from build123d import *

# Parameters (mm, degrees)
SKETCH1_R           = 88.9
SKETCH1_R_2         = 2.1
BOSS_EXTRUDE1_DEPTH = 6.35
SKETCH2_R           = 57.3
CUT_EXTRUDE1_DEPTH  = 3


with BuildPart() as part:
    # Sketch1 → Boss-Extrude1 (new, symmetric)
    with BuildSketch(Plane.XY):
        Circle(SKETCH1_R)
        with Locations((-12, 0)):
            Circle(SKETCH1_R_2, mode=Mode.SUBTRACT)
        with Locations((-6, 10.392304845)):
            Circle(SKETCH1_R_2, mode=Mode.SUBTRACT)
        with Locations((6, 10.392304845)):
            Circle(SKETCH1_R_2, mode=Mode.SUBTRACT)
        with Locations((12, 0)):
            Circle(SKETCH1_R_2, mode=Mode.SUBTRACT)
        with Locations((6, -10.392304845)):
            Circle(SKETCH1_R_2, mode=Mode.SUBTRACT)
        with Locations((-6, -10.392304845)):
            Circle(SKETCH1_R_2, mode=Mode.SUBTRACT)
    extrude(amount=BOSS_EXTRUDE1_DEPTH, both=True)

    # Sketch2 → Cut-Extrude1 (cut)
    with BuildSketch(Plane(origin=(0, 0, -6.35), x_dir=(-1, 0, 0), z_dir=(0, 0, -1))):
        Circle(SKETCH2_R)
    extrude(amount=-CUT_EXTRUDE1_DEPTH, mode=Mode.SUBTRACT)


solid = part.part
Design review of the part built by this model. Coordinates are the model's own, in mm. A direction names the side the tool comes from. Coordinates: 2 decimals unless noted, no trailing zeros. Write each loop counter-clockwise with the first axis right and the second up, starting at its lowest first coordinate (ties: lowest second). Pieces come first, ordered by that corner, then holes. Notation, with made-up numbers: (60, 46.5) - (101, 46.5) arc R11 cw to (101, 62.5) - close; hole circle Ø9 at (20, -9). An arc over 180 degrees is marked (long way). One line per item, written item: value.
1) Add section B-B (x = 0). State the section outline as (y, z) points.
Answer sheet:
outline: (-88.9, -6.35) - (-57.3, -6.35) - (-57.3, -3.35) - (57.3, -3.35) - (57.3, -6.35) - (88.9, -6.35) - (88.9, 6.35) - (-88.9, 6.35) - close
2) Insertion check: pin 1 (4 mm diameter, centred on y = 58.5, z = -3, fed in from +X); pin 2 (1.5 mm diameter, centred on y = -40, z = 2, fed in from -X); pin 3 (6 mm diameter, centred on x = 8, z = -2, fed in from -Y); pin 4 (5 mm diameter, centred on x = 12, y = 0, fed in from +Z). Each pin has a flat end and moves straight along its axis. Give the tip position at first contact, or say it passes through.
Answer sheet:
pin 1: stops at x = 68.64
pin 2: stops at x = -79.77
pin 3: stops at y = -88.76
pin 4: stops at z = 6.35
3) For faces 4 (the face through (-6.46, -12.44, 1.43)), 5 (the face through (1, 1, -3.35)), list the 3-axis set-ups (+Z, -Z, +X, -X, +Y, -Y) from which the entire face can be reached by the end or side of a thin tool; tool diameter is ignored.
Answer sheet:
face 4: +Z, -Z
face 5: -Z
4) Add section D-D (y = 32.5). State the section outline as (x, z) points, plus the area to 3 significant figures.
Answer sheet:
outline: (-82.75, -6.35) - (-47.19, -6.35) - (-47.19, -3.35) - (47.19, -3.35) - (47.19, -6.35) - (82.75, -6.35) - (82.75, 6.35) - (-82.75, 6.35) - close
area: 1,820 mm2
5) To check wall thickness, follow probe 1 along Y at (x, z) = (6, 2.5); probe 2 along X at (y, z) = (11, -2.5); probe 3 along Y at (x, z) = (-6.5, -2.25). State the ranges of each line that lie inside material, in increasing order.
Answer sheet:
probe 1: y = -88.7 to -12.49, -8.29 to 8.29, 12.49 to 88.7
probe 2: x = -88.22 to -8.01, -3.99 to 3.99, 8.01 to 88.22
probe 3: y = -88.66 to -12.43, -8.35 to 8.35, 12.43 to 88.66
6) Add section A-A (y = 0). State the section outline as (x, z) points, plus the area to 3 significant figures.
Answer sheet:
outline: (-88.9, -6.35) - (-57.3, -6.35) - (-57.3, -3.35) - (-14.1, -3.35) - (-14.1, 6.35) - (-88.9, 6.35) - close; (-9.9, -3.35) - (9.9, -3.35) - (9.9, 6.35) - (-9.9, 6.35) - close; (14.1, -3.35) - (57.3, -3.35) - (57.3, -6.35) - (88.9, -6.35) - (88.9, 6.35) - (14.1, 6.35) - close
area: 1,830 mm2
7) Mouldability with a two-part tool opening along X and no side actions: class faces 1 (the face through (-1, -58, -6.35)), 2 (the face through (84.795, 26.703, 0.089)), 3 (the face through (-6.273, 12.474, 1.432)) as +X half, -X half, draft (parallel to the pull), parting line (faces both ways), or undercut.
Answer sheet:
face 1: draft
face 2: parting line
face 3: undercut
8) Add section C-C (z = 1.25). State the section outline as (x, y) points.
Answer sheet:
outline: circle Ø177.8 at (0, 0); hole circle Ø4.2 at (-12, 0); hole circle Ø4.2 at (-6, -10.39); hole circle Ø4.2 at (-6, 10.39); hole circle Ø4.2 at (6, -10.39); hole circle Ø4.2 at (6, 10.39); hole circle Ø4.2 at (12, 0)
